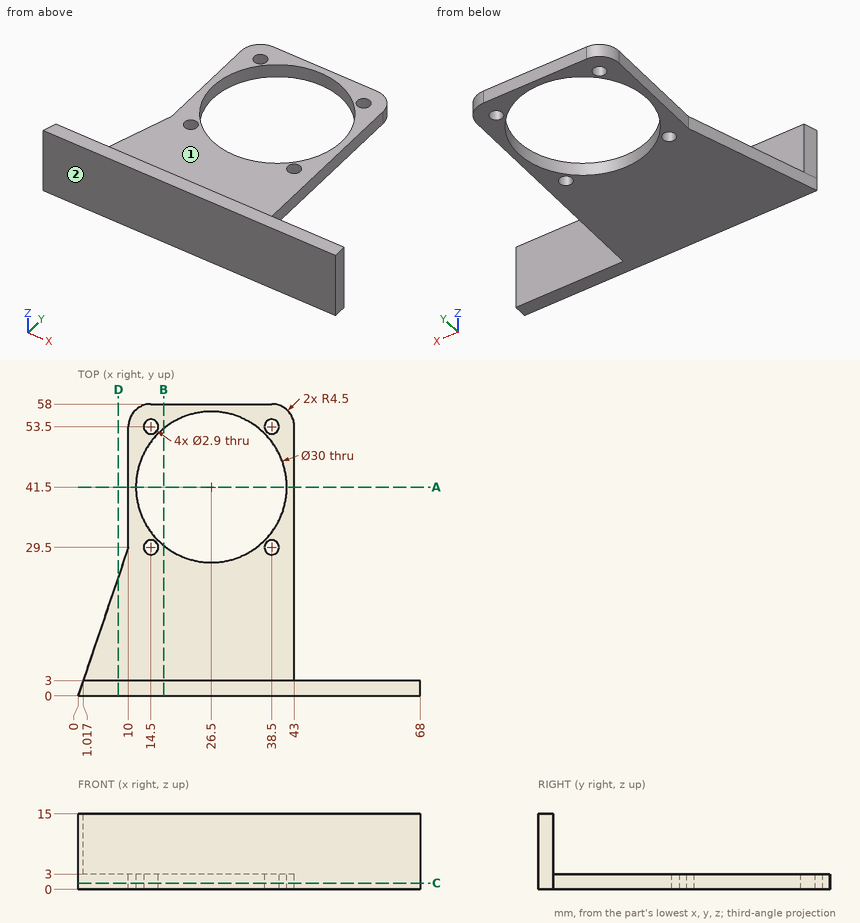
For this review, use the dimensioned drawing (mm, ordinates from the lowest corner) and the shaded views. A direction names the side the tool comes from. Coordinates: 2 decimals unless noted, no trailing zeros. Loops run counter-clockwise (first coordinate to the right, second up) from the corner with the lowest first, then second, coordinate; pieces in that order, holes last. Notation, with made-up numbers: (49, 27) -> (67, 27) arc R28 cw to (67, 59) -> close; hole circle Ø10 at (58.5, 20.25). An arc over 180 degrees is marked (long way). Use a Markdown table: item, result. Add a question column.
1. Clearance check with flat-ended pins moving along their axes: pin 1 Ø0.9 at (y, z) = (45, 2) entering from -X; pin 2 Ø4.5 at (x, y) = (14.5, 29.5) entering from -Z; pin 3 Ø3.5 at (x, y) = (14.5, 53.5) entering from +Z; pin 4 Ø1 at (x, z) = (11.5, 8.5) entering from +Y. State where each tip first meets the part, or that it passes through.
2. Add section D-D on x = 8. Write out the cut boundary in (y, z).
3. Add section A-A on y = 41.5. Write out the cut boundary in (x, z).
4. Add section C-C on z = 1.25. Write out the cut boundary in (x, y), plus the area to 3 significant figures.
5. Machinability: for the marked faces 1 and 2, which of the approach directions +Z, -Z, +X, -X, +Y, -Y give a long, thin tool a straight path to every point of the face, cutting with its end or side? Answer none if there is none.
6. To check wall thickness, follow line 1 (Y direction, x = 26.5, z = 1.05); line 2 (Y direction, x = 14.5, z = 0.95); line 3 (Y direction, x = 39, z = 12). State the ranges of each line that lie inside material, in increasing order.
7. Add section B-B on x = 17. Write out the cut boundary in (y, z), plus the area to 3 significant figures.
Returned:
| question | item | result |
|---|---|---|
| 1 | pin 1 | stops at x = 10 |
| 1 | pin 2 | stops at z = 0 |
| 1 | pin 3 | stops at z = 3 |
| 1 | pin 4 | stops at y = 3 |
| 2 | outline | (0, 0) -> (23.6, 0) -> (23.6, 3) -> (3, 3) -> (3, 15) -> (0, 15) -> close |
| 3 | outline | (10, 0) -> (11.5, 0) -> (11.5, 3) -> (10, 3) -> close; (41.5, 0) -> (43, 0) -> (43, 3) -> (41.5, 3) -> close |
| 4 | outline | (0, 0) -> (68, 0) -> (68, 3) -> (43, 3) -> (43, 53.5) arc R4.5 ccw to (38.5, 58) -> (14.5, 58) arc R4.5 ccw to (10, 53.5) -> (10, 29.5) -> close; hole circle Ø30 at (26.5, 41.5); hole circle Ø2.9 at (14.5, 29.5); hole circle Ø2.9 at (14.5, 53.5); hole circle Ø2.9 at (38.5, 29.5); hole circle Ø2.9 at (38.5, 53.5) |
| 4 | area | 1,390 mm² |
| 5 | face 1 | +Z, +X, -X, +Y |
| 5 | face 2 | +Z, -Z, +X, -X, -Y |
| 6 | line 1 | y = 0 to 26.5, 56.5 to 58 |
| 6 | line 2 | y = 0 to 28.05, 30.95 to 32.5, 50.5 to 52.05, 54.95 to 58 |
| 6 | line 3 | y = 0 to 3 |
| 7 | outline | (0, 0) -> (29.89, 0) -> (29.89, 3) -> (3, 3) -> (3, 15) -> (0, 15) -> close; (53.11, 0) -> (58, 0) -> (58, 3) -> (53.11, 3) -> close |
| 7 | area | 140 mm² |
